The model under review builds one solid part; all positions refer to its coordinate system, in mm. Give positions to 0.01 mm unless a question says otherwise; leave off trailing zeros. Loops run counter-clockwise (first coordinate to the right, second up) from the corner with the lowest first, then second, coordinate; pieces in that order, holes last. Notation, with made-up numbers: M 87.5,86.25 L 137.5,86.25 A29 ccw 137.5,109.25 Z; hole C 86.5,11 d1. An arc over 180 degrees is marked long. One line per item, written item: value. Start each with the question number.
Q1. We need section B-B on x = 60. Write out the cut boundary in (y, z), plus the area to 3 significant figures.
Q2. We need section C-C on z = 7.25. Write out the cut boundary in (x, y) (1 decimal).
Q3. For pin 1 (10 mm diameter, centred on x = 58.5, y = 72.5, fed in from -Z); pin 2 (6 mm diameter, centred on x = 51, y = 12.5, fed in from +Z), all flat-tipped, find the tip position at first contact; note any pin that passes through.
Q4. We need section D-D on x = 72.5. Write out the cut boundary in (y, z) (3 decimals).
Q5. We need section A-A on y = 41. Write out the cut boundary in (x, z).
Q6. To check wall thickness, follow line 1 along X through (y, z) = (79.5, 7); line 2 along Z through (x, y) = (69.5, 35.5). State the ranges of each line that lie inside material, in increasing order. Write a range as from..to.
```python
from build123d import *

# Parameters (mm, degrees)
SKETCH1_W           = 78.486
SKETCH1_H           = 86.614
BOSS_EXTRUDE1_DEPTH = 2.54
SKETCH2_R           = 1.5875
BOSS_EXTRUDE2_DEPTH = 9.525


with BuildPart() as part:
    # Sketch1 → Boss-Extrude1 (new body)
    with BuildSketch(Plane.XY):
        with Locations((39.243, 43.307)):
            Rectangle(SKETCH1_W, SKETCH1_H)
    extrude(amount=BOSS_EXTRUDE1_DEPTH)

    # Sketch2 → Boss-Extrude2 (add)
    with BuildSketch(Plane.XY.offset(2.54)):
        with Locations((6.223, 80.1116)):
            Circle(SKETCH2_R)
        with Locations((72.263, 80.1116)):
            Circle(SKETCH2_R)
        with Locations((72.263, 3.9116)):
            Circle(SKETCH2_R)
        with Locations((6.223, 3.9116)):
            Circle(SKETCH2_R)
    extrude(amount=BOSS_EXTRUDE2_DEPTH)


solid = part.part
```
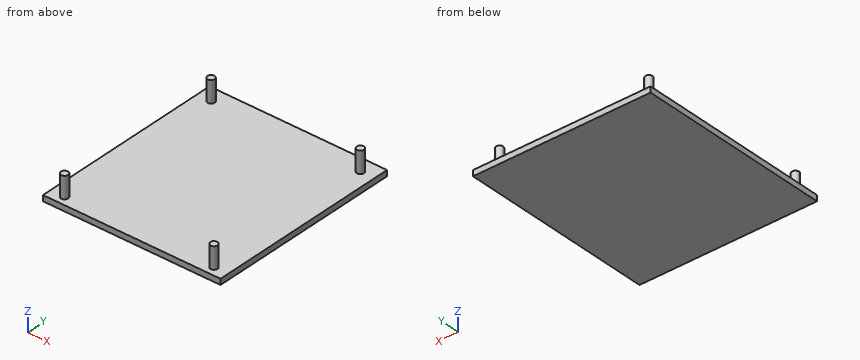
Solved:
1. outline: M 0,0 L 86.61,0 L 86.61,2.54 L 0,2.54 Z
1. area: 220 mm2
2. outline: C 6.2,3.9 d3.2; C 6.2,80.1 d3.2; C 72.3,3.9 d3.2; C 72.3,80.1 d3.2
3. pin 1: z = 0
3. pin 2: z = 2.54
4. outline: M 0,0 L 86.614,0 L 86.614,2.54 L 81.681,2.54 L 81.681,12.065 L 78.542,12.065 L 78.542,2.54 L 5.481,2.54 L 5.481,12.065 L 2.342,12.065 L 2.342,2.54 L 0,2.54 Z
5. outline: M 0,0 L 78.49,0 L 78.49,2.54 L 0,2.54 Z
6. line 1: 4.76..7.69, 70.8..73.73
6. line 2: 0..2.54
